The listing builds one solid part. Answer for the finished solid, in the listing's coordinates (mm). Coordinates: 2 decimals unless noted, no trailing zeros. Order: outer loops, then holes, each group sorted by start corner. A loop starts at its lowest first (then second) coordinate and runs counter-clockwise, first axis right, second up.
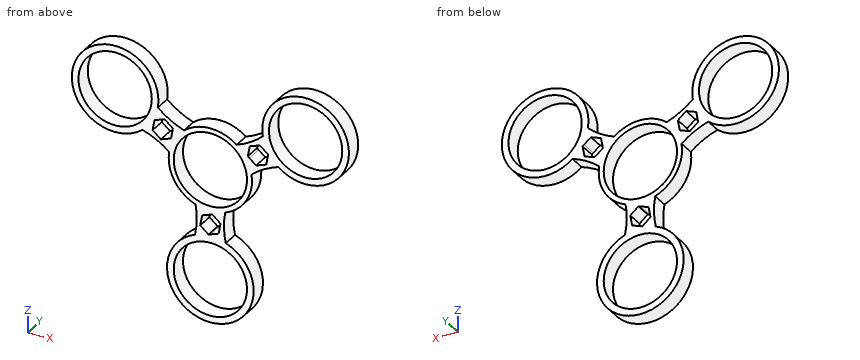
```python
from build123d import *

# Parameters (mm, degrees)
F0_R     = 11
F1_DEPTH = 5


with BuildPart() as f1:
    # F0 (on Front) → F1 (new body)
    with BuildSketch(Plane.XZ):
        with BuildLine():
            ThreePointArc((12.3414423693, 1.9846410874), (16.1365395854, 4.5999074354), (20.3716352974, 6.4182432847))
            ThreePointArc((20.3716352974, 6.4182432847), (39.8371685741, 23), (15.744179381, 14.4332320418))
            ThreePointArc((15.744179381, 14.4332320418), (12.0519064868, 11.6746994925), (7.8894707837, 9.6956820675))
            ThreePointArc((7.8894707837, 9.6956820675), (0, 12.5), (-7.8894707837, 9.6956820675))
            ThreePointArc((-7.8894707837, 9.6956820675), (-12.0519064868, 11.6746994925), (-15.744179381, 14.4332320418))
            ThreePointArc((-15.744179381, 14.4332320418), (-39.8371685741, 23), (-20.3716352974, 6.4182432847))
            ThreePointArc((-20.3716352974, 6.4182432847), (-16.1365395854, 4.5999074354), (-12.3414423693, 1.9846410874))
            ThreePointArc((-12.3414423693, 1.9846410874), (-10.8253175473, -6.25), (-4.4519715856, -11.6803231548))
            ThreePointArc((-4.4519715856, -11.6803231548), (-4.0846330986, -16.2746069278), (-4.6274559164, -20.8514753266))
            ThreePointArc((-4.6274559164, -20.8514753266), (0, -46), (4.6274559164, -20.8514753266))
            ThreePointArc((4.6274559164, -20.8514753266), (4.0846330986, -16.2746069278), (4.4519715856, -11.6803231548))
            ThreePointArc((4.4519715856, -11.6803231548), (10.8253175473, -6.25), (12.3414423693, 1.9846410874))
        make_face()
        with Locations((0, -33)):
            Circle(F0_R, mode=Mode.SUBTRACT)
        Polygon((0.5784799381, -13.3175262717), (3.0453430646, -15.4097414578), (2.4668631266, -18.5922151861), (0, -19.4753730239), (-0.5784799381, -19.6824737283), (-3.0453430646, -17.5902585422), (-2.4668631266, -14.4077848139), (0, -13.5246269761), align=None, mode=Mode.SUBTRACT)
        Polygon((-11.8225560359, 6.1577848139), (-14.8678991005, 5.0675262717), (-17.3347622271, 7.1597414578), (-16.756282289, 10.3422151861), (-13.7109392244, 11.4324737283), (-11.2440760978, 9.3402585422), align=None, mode=Mode.SUBTRACT)
        with Locations((-28.5788383249, 16.5)):
            Circle(F0_R, mode=Mode.SUBTRACT)
        Circle(F0_R, mode=Mode.SUBTRACT)
        Polygon((17.3347622271, 9.3402585422), (16.756282289, 6.1577848139), (13.7109392244, 5.0675262717), (11.712670538, 6.7623134881), (11.2440760978, 7.1597414578), (11.8225560359, 10.3422151861), (14.8678991005, 11.4324737283), (16.8661677868, 9.7376865119), align=None, mode=Mode.SUBTRACT)
        with Locations((28.5788383249, 16.5)):
            Circle(F0_R, mode=Mode.SUBTRACT)
    extrude(amount=F1_DEPTH)


solid = f1.part
```
1) A cutting plane is placed at A-A, the plane z = -33. Write down the section's boundary in (x, y).
2) A cutting plane is placed at D-D, the plane y = -2.7. Count the separate pieces of the cut face and the enclosed holes in it, plus the area to 3 significant figures.
3) A cutting plane is placed at C-C, the plane x = 34. Write down the section's boundary in (y, z), plus the area to 3 significant figures.
4) Each of these flat-tipped pins is pushed along its axis until it touches: P1, Ø2, axis at x = 3, y = -2, coming from the +Z side; P2, Ø3, axis at y = -3.5, z = -32, coming from the +X side; P3, Ø17.5, axis at x = 28.58, z = 16.5, coming from the +Y side. Where does it stop, or does it pass through?
5) A cutting plane is placed at B-B, the plane z = 16.5. Write down the section's boundary in (x, y), plus the area to 3 significant figures.
6) Straight lines are drawn through the part: probe 1 along Z at (x, y) = (10, -2.4); probe 2 along X at (y, z) = (-1.45, 5); probe 3 along Z at (x, y) = (31, -0.4). For each, find the intervals that lie inside material, in ascending order.
Working result:
1. outline: (-13, -5) - (-11, -5) - (-11, 0) - (-13, 0) - close; (11, -5) - (13, -5) - (13, 0) - (11, 0) - close
2. separate pieces: 1
2. enclosed holes: 7
2. area: 684 mm2
3. outline: (-5, 4.68) - (0, 4.68) - (0, 6.93) - (-5, 6.93) - close; (-5, 26.07) - (0, 26.07) - (0, 28.32) - (-5, 28.32) - close
3. area: 22.4 mm2
4. P1: stops at z = 12.34
4. P2: stops at x = 13
4. P3: passes through
5. outline: (-41.58, -5) - (-39.58, -5) - (-39.58, 0) - (-41.58, 0) - close; (-17.58, -5) - (-15.58, -5) - (-15.58, 0) - (-17.58, 0) - close; (15.58, -5) - (17.58, -5) - (17.58, 0) - (15.58, 0) - close; (39.58, -5) - (41.58, -5) - (41.58, 0) - (39.58, 0) - close
5. area: 40.0 mm2
6. probe 1: z = -41.31 to -37.58, -28.42 to -24.69, -7.5 to -4.58, 4.58 to 10.57
6. probe 2: x = -34.64 to -22.52, -16.89 to -9.8, 9.8 to 16.89, 22.52 to 34.64
6. probe 3: z = 3.73 to 5.77, 27.23 to 29.27
